from build123d import *

# Parameters (mm, degrees)
F0_R     = 13.5
F1_DEPTH = 24.5
F2_R     = 2.5
F3_DEPTH = 14
F5_DEPTH = 5
F6_SIZE  = 1
F7_SIZE  = 4


with BuildPart() as f1:
    # F0 (on Top) → F1 (new body)
    with BuildSketch(Plane.XY):
        Circle(F0_R)
    extrude(amount=F1_DEPTH)

    # F2 (on face) → F3 (join)
    with BuildSketch(Plane.XY.offset(24.5)):
        Circle(F2_R)
    extrude(amount=F3_DEPTH)

    # F4 (on face) → F5 (cut)
    with BuildSketch(Plane(origin=(0, 0, 0), x_dir=(1, 0, 0), z_dir=(0, 0, -1))):
        with BuildLine():
            ThreePointArc((8.217514, -6.717514), (7.29154, -5.331695), (5.656854, -5.656854))
            ThreePointArc((5.656854, -5.656854), (6.143489, -8.103334), (8.217514, -6.717514))
        make_face()
        with BuildLine():
            ThreePointArc((-5.217514, 6.717514), (-8.103334, 7.29154), (-5.656854, 5.656854))
            ThreePointArc((-5.656854, 5.656854), (-5.331695, 6.143489), (-5.217514, 6.717514))
        make_face()
        with BuildLine():
            ThreePointArc((7.156854, 5.656854), (5.082829, 7.042674), (4.596194, 4.596194))
            ThreePointArc((4.596194, 4.596194), (6.230879, 4.271035), (7.156854, 5.656854))
        make_face()
        with BuildLine():
            ThreePointArc((-4.156854, -5.656854), (-4.271035, -5.082829), (-4.596194, -4.596194))
            ThreePointArc((-4.596194, -4.596194), (-7.042674, -6.230879), (-4.156854, -5.656854))
        make_face()
    extrude(amount=-F5_DEPTH, mode=Mode.SUBTRACT)

    # F6
    f6_edges = [f1.edges().sort_by_distance(p)[0] for p in [
        (-13.5, 0, 0),
    ]]
    chamfer(f6_edges, length=F6_SIZE)

    # F7
    f7_edges = [f1.edges().sort_by_distance(p)[0] for p in [
        (-13.5, 0, 24.5),
    ]]
    chamfer(f7_edges, length=F7_SIZE)


solid = f1.part
Can you work these out from the model? Positions are in its coordinate system, mm. A direction names the side the tool comes from. Coordinates: 2 decimals unless noted, no trailing zeros. Loops run counter-clockwise (first coordinate to the right, second up) from the corner with the lowest first, then second, coordinate; pieces in that order, holes last. Notation, with made-up numbers: (21.25, -5.75) - (47.25, -5.75) arc R12 cw to (47.25, -0.75) - close; hole circle Ø7 at (22.5, 40.25). An arc over 180 degrees is marked (long way). Put each result on its own line as item: value. Start each with the question number.
Item 1: If we mould it in two halves opening along Y, with no side actions, what happens to faces 1 (the face through (9.247, 2.912, 24.306)), 2 (the face through (0, 0, 38.5)), 3 (the face through (-7, -7, 5))? For each: +Y half, -Y half, draft (parallel to the pull), parting line (faces both ways), or undercut.
Item 2: Which directions (+Z, -Z, +X, -X, +Y, -Y) give clear straight access to the entire face, cutting with the end or side of a thin tool? Please do faces 4 (the face through (-6, 6, 5)), 5 (the face through (0, 0, 0)), 6 (the face through (2, -2, 24.5)).
Item 3: If I drill on line 1 along Y through (x, z) = (-6, 4.5); line 2 along Y through (x, z) = (0, 5), over which ranges is the centre line in solid material (lowest first)?
Item 4: Suppose I cut it at A-A (x = 0). Please give me the cut outline in (y, z).
Item 5: For pin 1 (8 mm diameter, centred on x = -8.5, z = 23.5, fed in from -Y); pin 2 (0.9 mm diameter, centred on x = -6, y = 5.5, fed in from -Z); pin 3 (2 mm diameter, centred on x = 1, y = 10.5, fed in from +Z), each with a flat end and sliding along its axis, tell me the tip position at first contact or that it passes through.
Item 6: Suppose I cut it at D-D (z = 23.5). Please give me the cut outline in (x, y).
Item 7: Suppose I cut it at C-C (z = 8). Please give me the cut outline in (x, y).
Here are the results:
1. face 1: parting line
1. face 2: draft
1. face 3: undercut
2. face 4: -Z
2. face 5: -Z, +X, -X, +Y, -Y
2. face 6: +Z
3. line 1: -12.09 to -8.03, -5.4 to 4.2, 7.12 to 12.09
3. line 2: -13.5 to 13.5
4. outline: (-13.5, 1) - (-12.5, 0) - (12.5, 0) - (13.5, 1) - (13.5, 20.5) - (9.5, 24.5) - (2.5, 24.5) - (2.5, 38.5) - (-2.5, 38.5) - (-2.5, 24.5) - (-9.5, 24.5) - (-13.5, 20.5) - close
5. pin 1: y = -12.16
5. pin 2: z = 5
5. pin 3: z = 24.45
6. outline: circle Ø21 at (0, 0)
7. outline: circle Ø27 at (0, 0)
